from build123d import *

# Parameters (mm, degrees)
SKETCH1_W                    = 20.32
SKETCH1_H                    = 55.88
BASE_FLANGE1_DEPTH           = 2.286
EDGE_FLANGE1_STRIP_W         = 10.144
EDGE_FLANGE1_STRIP_H         = 2.286
EDGE_FLANGE1_STRIP_CUT_DEPTH = 20.32
EDGE_FLANGE1_DEPTH           = 20.32
SKETCH9_R                    = 3.05
CUT_EXTRUDE1_DEPTH           = 79.090440106
SKETCH10_R                   = 3.05
SKETCH10_R_2                 = 1.75
CUT_EXTRUDE2_DEPTH           = 62.287731529


# Sheet-metal steps are written as plain solids
with BuildPart() as part:
    # Sketch1 → Base-Flange1 (new body)
    with BuildSketch(Plane(origin=(0, 0, 0), x_dir=(1, 0, 0), z_dir=(0, 1, 0))):
        Rectangle(SKETCH1_W, SKETCH1_H)
    extrude(amount=-BASE_FLANGE1_DEPTH)

    # Edge-Flange1 strip (across the edge) → Edge-Flange1 strip cut (cut)
    with BuildSketch(Plane(origin=(10.16, 0, -27.94), x_dir=(0, 0, 1), z_dir=(-1, 0, 0))):
        with Locations((-2.286, -1.143)):
            Rectangle(EDGE_FLANGE1_STRIP_W, EDGE_FLANGE1_STRIP_H)
    extrude(amount=EDGE_FLANGE1_STRIP_CUT_DEPTH, mode=Mode.SUBTRACT)

    # Edge-Flange1 section (across the edge) → Edge-Flange1 (add)
    with BuildSketch(Plane(origin=(10.16, 0, -27.94), x_dir=(0, 0, 1), z_dir=(-1, 0, 0))):
        with BuildLine():
            Line((0, 0.5), (0, 53.594))
            Line((0, 53.594), (2.286, 53.594))
            Line((2.286, 53.594), (2.286, 0.5))
            ThreePointArc((2.286, 0.5), (2.432446609, 0.146446609), (2.786, 0))
            Line((2.786, 0), (2.786, -2.286))
            ThreePointArc((2.786, -2.286), (0.816000508, -1.469999492), (0, 0.5))
        make_face()
    extrude(amount=EDGE_FLANGE1_DEPTH)

    # Sketch9 → Cut-Extrude1 (cut, through all)
    with BuildSketch(Plane(origin=(0, 0, -27.94), x_dir=(-1, 0, 0), z_dir=(0, 0, -1))):
        with Locations(Location((0, 35.695518005, 0), (0, 0, 90))):
            Circle(SKETCH9_R)
        with BuildLine():
            ThreePointArc((-5.020458146, 42.465976152), (-6.770458146, 40.715976152), (-5.020458146, 38.965976152))
            ThreePointArc((-5.020458146, 38.965976152), (-3.270458146, 40.715976152), (-5.020458146, 42.465976152))
        make_face()
        with BuildLine():
            ThreePointArc((-5.020458146, 32.425059859), (-6.770458146, 30.675059859), (-5.020458146, 28.925059859))
            ThreePointArc((-5.020458146, 28.925059859), (-3.270458146, 30.675059859), (-5.020458146, 32.425059859))
        make_face()
        with BuildLine():
            ThreePointArc((5.020458146, 32.425059859), (3.270458146, 30.675059859), (5.020458146, 28.925059859))
            ThreePointArc((5.020458146, 28.925059859), (6.770458146, 30.675059859), (5.020458146, 32.425059859))
        make_face()
        with BuildLine():
            ThreePointArc((5.020458146, 42.465976152), (3.270458146, 40.715976152), (5.020458146, 38.965976152))
            ThreePointArc((5.020458146, 38.965976152), (6.770458146, 40.715976152), (5.020458146, 42.465976152))
        make_face()
    extrude(amount=-CUT_EXTRUDE1_DEPTH, mode=Mode.SUBTRACT)

    # Sketch10 → Cut-Extrude2 (cut, through all)
    with BuildSketch(Plane(origin=(0, 0, 0), x_dir=(1, 0, 0), z_dir=(0, 1, 0))):
        with Locations(Location((-0.01000002, -1.426000002, 0), (0, 0, 270))):
            Circle(SKETCH10_R)
        with Locations(Location((-5.030458167, -16.487374441, 0), (0, 0, 270))):
            Circle(SKETCH10_R_2)
        with Locations(Location((-5.030458167, 3.594458144, 0), (0, 0, 270))):
            Circle(SKETCH10_R_2)
        with Locations(Location((5.010458126, 13.635374437, 0), (0, 0, 270))):
            Circle(SKETCH10_R_2)
        with Locations(Location((5.010458126, -6.446458149, 0), (0, 0, 270))):
            Circle(SKETCH10_R_2)
        with Locations(Location((5.010458126, -16.487374441, 0), (0, 0, 270))):
            Circle(SKETCH10_R_2)
        with Locations(Location((-5.030458167, 13.635374437, 0), (0, 0, 270))):
            Circle(SKETCH10_R_2)
        with Locations(Location((-5.030458167, -6.446458149, 0), (0, 0, 270))):
            Circle(SKETCH10_R_2)
        with Locations(Location((5.010458126, 3.594458144, 0), (0, 0, 270))):
            Circle(SKETCH10_R_2)
    extrude(amount=-CUT_EXTRUDE2_DEPTH, mode=Mode.SUBTRACT)


solid = part.part
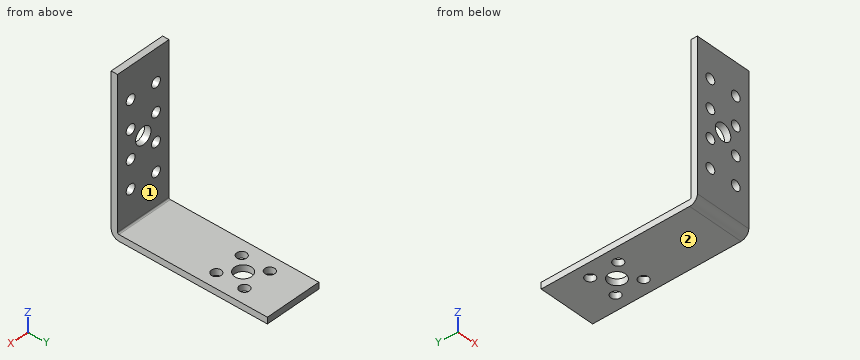
Work out the finished part from the listing and answer in its coordinate system (mm). Face numbers are marked on the shaded views. A direction names the side the tool comes from. Give positions to 0.01 mm unless a question says otherwise; leave off trailing zeros. Loops run counter-clockwise (first coordinate to the right, second up) from the corner with the lowest first, then second, coordinate; pieces in that order, holes last. Notation, with made-up numbers: (49, 79.5) -> (65, 79.5) arc R25 ccw to (65, 93.5) -> close; hole circle Ø2 at (83, 7.25). An arc over 180 degrees is marked (long way). Use a Markdown table: item, result. Add a question column.
1) The part is cut by section A-A, the plane x = -0.75. Determine the outline of the cut face in (y, z), plus the area to 3 significant figures.
2) Which of the six approach directions +Z, -Z, +X, -X, +Y, -Y give full straight-line access (tool end or side, diameter ignored) to the marked faces 1 and 2?
3) The part is cut by section B-B, the plane z = 2. Determine the outline of the cut face in (x, y), plus the area to 3 significant figures.
4) Consider line 1 along Y through (x, z) = (-0.25, 23); line 2 along Z through (x, y) = (5.75, 8). Determine where each line is inside the solid, lowest interval first.
5) Each of these flat-tipped pins is pushed along its axis until it touches: P1, Ø4.5, axis at x = -5.03, z = 6.45, coming from the +Y side; P2, Ø5, axis at x = 0, y = 35.7, coming from the +Z side; P3, Ø6, axis at x = -3, y = 29.5, coming from the +Z side. Where does it stop, or does it pass through?
6) The part is cut by section D-D, the plane y = 48. Determine the outline of the cut face in (x, z).
7) The part is cut by section C-C, the plane x = 4.25. Count the separate pieces of the cut face and the enclosed holes in it, plus the area to 3 significant figures.
Reported:
| question | item | result |
|---|---|---|
| 1 | outline | (-2.29, -25.15) arc R2.79 ccw to (0.5, -27.94) -> (32.74, -27.94) -> (32.74, -25.65) -> (0.5, -25.65) arc R0.5 cw to (0, -25.15) -> (0, -1.53) -> (-2.29, -1.53) -> close; (-2.29, 4.38) -> (0, 4.38) -> (0, 27.94) -> (-2.29, 27.94) -> close; (38.65, -27.94) -> (53.59, -27.94) -> (53.59, -25.65) -> (38.65, -25.65) -> close |
| 1 | area | 222 mm^2 |
| 2 | face 1 | +Z, +X, -X, +Y |
| 2 | face 2 | -Z, +X, -X, +Y, -Y |
| 3 | outline | (-10.16, -2.29) -> (-3.01, -2.29) -> (-3.01, 0) -> (-10.16, 0) -> close; (2.99, -2.29) -> (10.16, -2.29) -> (10.16, 0) -> (2.99, 0) -> close |
| 3 | area | 32.8 mm^2 |
| 4 | line 1 | y = -2.29 to 0 |
| 4 | line 2 | z = -27.94 to -25.65 |
| 5 | P1 | stops at y = 0 |
| 5 | P2 | passes through |
| 5 | P3 | stops at z = -25.65 |
| 6 | outline | (-10.16, -27.94) -> (10.16, -27.94) -> (10.16, -25.65) -> (-10.16, -25.65) -> close |
| 7 | separate pieces | 7 |
| 7 | enclosed holes | 0 |
| 7 | area | 205 mm^2 |
